Design review of the part built by this model. Coordinates are the model's own, in mm. A direction names the side the tool comes from. Round coordinates to 2 decimals unless told otherwise and drop trailing zeros. Loops run counter-clockwise (first coordinate to the right, second up) from the corner with the lowest first, then second, coordinate; pieces in that order, holes last. Notation, with made-up numbers: (-32, -22) -> (10, -22) arc R12 cw to (10, -3) -> close; hole circle Ø7 at (79, 27). An arc over 180 degrees is marked (long way). Answer as CSV lines item,"result". Start each with the question number.
(1) For P1, Ø0.5, axis at y = -0.5, z = 3, coming from the +X side; P2, Ø1.5, axis at x = -8, y = -0.5, coming from the -Z side; P3, Ø1, axis at y = -0.5, z = -1.5, coming from the -X side; P4, Ø4.5, axis at x = -15, z = 0, coming from the +Y side, all flat-tipped, find the tip position at first contact; note any pin that passes through.
(2) Take a section at B-B, the plane x = 0. Write out the cut boundary in (y, z), and give its area (3 significant figures).
(3) To check wall thickness, follow line 1 (X direction, y = 0.8, z = 0); line 2 (X direction, y = 1.4, z = -4); line 3 (X direction, y = -1.4, z = -5.25). State the ranges of each line that lie inside material, in increasing order. Write a range as from..to.
(4) Take a section at D-D, the plane x = 5.5. Write out the cut boundary in (y, z), and give its area (3 significant figures).
(5) Take a section at A-A, the plane z = 0. Write out the cut boundary in (x, y).
(6) Take a section at C-C, the plane x = -15. Write out the cut boundary in (y, z), and give its area (3 significant figures).
(7) Machinability: for faces 1 (the face through (18.07, -0.03, 2.32)), 2 (the face through (-19.39, 0.03, 5.22)), which of the approach directions +Z, -Z, +X, -X, +Y, -Y give a long, thin tool a straight path to every point of the face, cutting with its end or side? Answer none if there is none.
(8) Draft analysis for pull direction X (two halves, no side actions). For faces 3 (the face through (0, 2, -6)), 4 (the face through (10.543, 0.028, 5.242)), state which applies: +X half, -X half, draft (parallel to the pull), parting line (faces both ways), or undercut.
from build123d import *

# Parameters (mm, degrees)
SKIZZE1_R                       = 3.75
AUFSATZ_LINEAR_AUSTRAGEN1_DEPTH = 2
SKIZZE2_R                       = 1.5
SCHNITT_LINEAR_AUSTRAGEN1_DEPTH = 25.677925359
VERRUNDUNG1_R                   = 2
VERRUNDUNG2_R                   = 2
SKIZZE4_R                       = 7.508546114
AUFSATZ_LINEAR_AUSTRAGEN2_DEPTH = 4
SKIZZE5_R                       = 4.5
SCHNITT_LINEAR_AUSTRAGEN3_DEPTH = 25.6779255
VERRUNDUNG4_R                   = 1


with BuildPart() as part:
    # Skizze1 → Aufsatz-Linear austragen1 (new, symmetric)
    with BuildSketch(Plane(origin=(0, 0, 0), x_dir=(1, 0, 0), z_dir=(0, 1, 0))):
        with BuildLine():
            Line((-7.583801513, -3), (0, -3))
            Line((0, -3), (0, 4))
            Line((0, 4), (-8.07179677, 4))
            ThreePointArc((-8.07179677, 4), (-22.980630624, -0.556358556), (-7.583801513, -3))
        make_face()
        with Locations(Location((-15, 0, 0), (0, 0, 270))):
            Circle(SKIZZE1_R, mode=Mode.SUBTRACT)
    extrude(amount=AUFSATZ_LINEAR_AUSTRAGEN1_DEPTH, both=True)

    # Skizze2 → Schnitt-Linear austragen1 (cut, through all)
    with BuildSketch(Plane(origin=(0, 2, 0), x_dir=(1, 0, 0), z_dir=(0, 1, 0))):
        with Locations((-8.07179677, 4)):
            Circle(SKIZZE2_R)
        with BuildLine():
            Line((-12, 0), (-12, -8))
            ThreePointArc((-12, -8), (-15, -11), (-18, -8))
            Line((-18, -8), (-18, 0))
            ThreePointArc((-18, 0), (-15, 3), (-12, 0))
        make_face()
    extrude(amount=-SCHNITT_LINEAR_AUSTRAGEN1_DEPTH, mode=Mode.SUBTRACT)

    # Verrundung1
    verrundung1_edges = [part.edges().sort_by_distance(p)[0] for p in [
        (-8.94027842, 0, -5.223004343),
        (-6.57179677, 0, -4),
        (-18, 0, 2.25),
        (-12, 0, 2.25),
        (-7.583801513, 0, 3),
    ]]
    fillet(verrundung1_edges, radius=VERRUNDUNG1_R)

    # Verrundung2
    verrundung2_edges = [part.edges().sort_by_distance(p)[0] for p in [
        (-12, 0, 7.416198487),
        (-18, 0, 7.416198487),
    ]]
    fillet(verrundung2_edges, radius=VERRUNDUNG2_R)

    # Spiegeln1: part across plane


with BuildPart() as part_1:
    add(part.part)
    add(part.part.mirror(Plane(origin=(0, 2, -4), x_dir=(0, 0, 1), z_dir=(-1, 0, 0))))

    # Skizze4 → Aufsatz-Linear austragen2 (add)
    with BuildSketch(Plane(origin=(0, 2, 0), x_dir=(1, 0, 0), z_dir=(0, 1, 0))):
        Circle(SKIZZE4_R)
    extrude(amount=-AUFSATZ_LINEAR_AUSTRAGEN2_DEPTH)

    # Skizze5 → Schnitt-Linear austragen3 (cut, through all)
    with BuildSketch(Plane(origin=(0, 2, 0), x_dir=(1, 0, 0), z_dir=(0, 1, 0))):
        with Locations(Location((0, 0, 0), (0, 0, 270))):
            Circle(SKIZZE5_R)
    extrude(amount=-SCHNITT_LINEAR_AUSTRAGEN3_DEPTH, mode=Mode.SUBTRACT)

    # Verrundung4
    verrundung4_edges = [part_1.edges().sort_by_distance(p)[0] for p in [
        (6.853540925, 0, 3.06712268),
        (-6.853540925, 0, 3.06712268),
    ]]
    fillet(verrundung4_edges, radius=VERRUNDUNG4_R)


solid = part_1.part
The answers:
1,P1,"x = 22.51"
1,P2,"z = -2.75"
1,P3,"x = -22.94"
1,P4,"through"
2,outline,"(-2, -7.51) -> (2, -7.51) -> (2, -4.5) -> (-2, -4.5) -> close; (-2, 4.5) -> (2, 4.5) -> (2, 7.51) -> (-2, 7.51) -> close"
2,area,"24.1 mm²"
3,line 1,"-23..-18.75, -11.25..-4.5, 4.5..11.25, 18.75..23"
3,line 2,"-21.93..-9.57, -6.35..-2.06, 2.06..6.35, 9.57..21.93"
3,line 3,"-21.04..-9.51, -5.37..5.37, 9.51..21.04"
4,outline,"(-2, -5.11) -> (2, -5.11) -> (2, 5.11) -> (-2, 5.11) -> close"
4,area,"40.9 mm²"
5,outline,"(-23, -2) -> (-18.75, -2) -> (-18.75, 2) -> (-23, 2) -> close; (-11.25, -2) -> (-4.5, -2) -> (-4.5, 2) -> (-11.25, 2) -> close; (4.5, -2) -> (11.25, -2) -> (11.25, 2) -> (4.5, 2) -> close; (18.75, -2) -> (23, -2) -> (23, 2) -> (18.75, 2) -> close"
6,outline,"(-2, -8) -> (2, -8) -> (2, -3.75) -> (-2, -3.75) -> close"
6,area,"17.0 mm²"
7,face 1,"+Y, -Y"
7,face 2,"+Z, +Y, -Y"
8,face 3,"draft"
8,face 4,"undercut"
